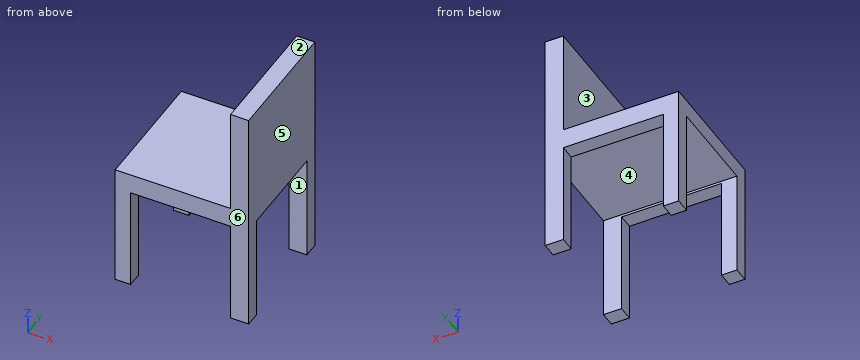
```python
from build123d import *

# Parameters (mm, degrees)
F1_DEPTH = 420
F2_W     = 320
F2_H     = 360
F3_DEPTH = 450.001


with BuildPart() as f1:
    # F0 (on Front) → F1 (new body)
    with BuildSketch(Plane.XZ):
        Polygon((0, 420), (0, 0), (51.913477, 0), (51.913477, 351.713803), (388.899834, 351.713803), (388.899834, 0), (450, 0), (450, 780), (388.899834, 780), (388.899834, 420), align=None)
    extrude(amount=F1_DEPTH)

    # F2 (on face) → F3 (cut, through all)
    with BuildSketch(Plane(origin=(0, 0, 0), x_dir=(0, -1, 0), z_dir=(-1, 0, 0))):
        with Locations((210, 180)):
            Rectangle(F2_W, F2_H)
    extrude(amount=-F3_DEPTH, mode=Mode.SUBTRACT)


solid = f1.part
```
The listing builds one solid part. Answer for the finished solid, in the listing's coordinates (mm). Face numbers are marked on the shaded views. A direction names the side the tool comes from. Round coordinates to 2 decimals unless told otherwise and drop trailing zeros. Loops run counter-clockwise (first coordinate to the right, second up) from the corner with the lowest first, then second, coordinate; pieces in that order, holes last. Notation, with made-up numbers: (5, -18) - (51, -18) arc R17 cw to (51, 13) - close; hole circle Ø1 at (36, 68). An arc over 180 degrees is marked (long way). Use one line per item in the form item = value. Start each with the question number.
1. The part is cut by section A-A on z = 96. Determine the outline of the cut face in (x, y), then the cut area to 3 significant figures.
2. A tool of negligible diameter and unlimited length cuts with its end or side. For the marked faces 1, 2 and 3, from which of +Z, -Z, +X, -X, +Y, -Y can it reach the whole face along a straight path? Write none if from no direction.
3. Consider line 1 (Z direction, x = 362.5, y = -338); line 2 (X direction, y = -394, z = 262); line 3 (X direction, y = -92, z = 682.5). Determine where each line is inside the solid, lowest interval first. Write a range as [from, to].
4. For a pull along Y with two mould halves and no side action, classify the marked faces 4, 5 and 6 as pulls with the +Y half, pulls with the -Y half, needs draft (parallel to the pull), parting line crosses it, or undercut.
5. The part is cut by section C-C on y = -204. Determine the outline of the cut face in (x, z).
6. The part is cut by section B-B on x = 32. Determine the outline of the cut face in (y, z).
7. The part is cut by section D-D on z = 684. Determine the outline of the cut face in (x, y), then the cut area to 3 significant figures.
8. Given pin 1 Ø2 at (x, y) = (342, -184) entering from -Z; pin 2 Ø1 at (y, z) = (-275.5, 635) entering from -X; pin 3 Ø25 at (x, y) = (288, -390) entering from -Z, each flat-ended and moving along its own axis, determine where each tip first touches the part or whether it passes through.
Geometry check:
q1.outline = (0, -420) - (51.91, -420) - (51.91, -370) - (0, -370) - close; (0, -50) - (51.91, -50) - (51.91, 0) - (0, 0) - close; (388.9, -420) - (450, -420) - (450, -370) - (388.9, -370) - close; (388.9, -50) - (450, -50) - (450, 0) - (388.9, 0) - close
q1.area = 11,300 mm^2
q2.face_1 = -Z, +X, -X
q2.face_2 = +Z, +X, -X, +Y, -Y
q2.face_3 = +Z, -X, +Y, -Y
q3.line_1 = [360, 420]
q3.line_2 = [0, 51.91], [388.9, 450]
q3.line_3 = [388.9, 450]
q4.face_4 = undercut
q4.face_5 = needs draft
q4.face_6 = pulls with the -Y half
q5.outline = (0, 360) - (450, 360) - (450, 780) - (388.9, 780) - (388.9, 420) - (0, 420) - close
q6.outline = (-420, 0) - (-370, 0) - (-370, 360) - (-50, 360) - (-50, 0) - (0, 0) - (0, 420) - (-420, 420) - close
q7.outline = (388.9, -420) - (450, -420) - (450, 0) - (388.9, 0) - close
q7.area = 25,700 mm^2
q8.pin_1 = 360
q8.pin_2 = 388.9
q8.pin_3 = 351.71
